Check sheet for the modelled part. Datum: model origin and axes. Units: mm. Face numbers are marked on the shaded views. Give positions to 0.01 mm unless a question says otherwise; leave off trailing zeros. Write each loop counter-clockwise with the first axis right and the second up, starting at its lowest first coordinate (ties: lowest second). Pieces come first, ordered by that corner, then holes.
from build123d import *

# Parameters (mm, degrees)
SKETCH1_W           = 105
SKETCH1_H           = 50
BOSS_EXTRUDE1_DEPTH = 5
BOSS_EXTRUDE2_DEPTH = 5


with BuildPart() as part:
    # Sketch1 → Boss-Extrude1 (new body)
    with BuildSketch(Plane(origin=(0, 0, 0), x_dir=(1, 0, 0), z_dir=(0, 1, 0))):
        Rectangle(SKETCH1_W, SKETCH1_H)
    extrude(amount=BOSS_EXTRUDE1_DEPTH)

    # Sketch2 → Boss-Extrude2 (add)
    with BuildSketch(Plane(origin=(0, 5, 0), x_dir=(1, 0, 0), z_dir=(0, 1, 0))):
        Polygon((-52.5, 25), (-52.5, -25), (52.5, -25), (52.5, 25), (47.5, 25), (47.5, -20), (-47.5, -20), (-47.5, 25), align=None)
    extrude(amount=BOSS_EXTRUDE2_DEPTH)


solid = part.part
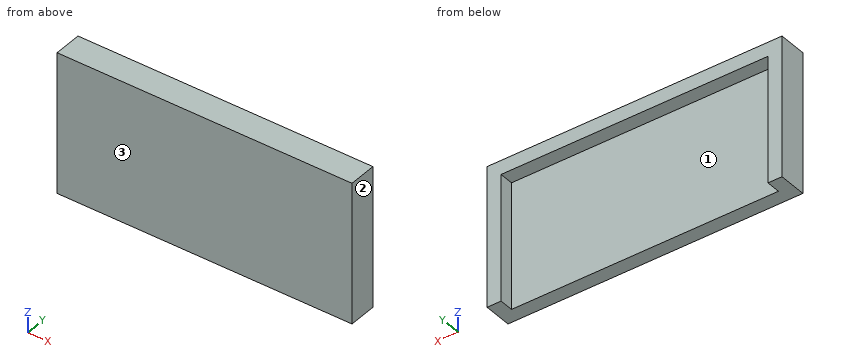
1) Draft check along X on the marked faces 1, 2 and 3. Enter one of: +X half, -X half, draft (parallel to the pull), parting line (faces both ways), or undercut.
2) Sectioned sample at B-B on y = 6. Record the boundary of the cut face in (x, z), then the cut area to 3 significant figures.
3) Scan lines: L1, parallel to X at y = 6, z = -5; L2, parallel to Z at x = -44, y = 6; L3, parallel to Y at x = 11.5, z = -15.5. Record each from-to range of solid material in increasing order.
4) Sectioned sample at C-C on x = 19. Record the boundary of the cut face in (y, z), then the cut area to 3 significant figures.
5) Gauge pin test, flat end, axial feed: pin 1 (13.5 mm diameter, centred on x = -15.5, z = -4.5, fed in from +Y). Record the tip position at first contact, or that the pin passes through.
6) Sectioned sample at A-A on z = -10.5. Record the boundary of the cut face in (x, y).
Answers below:
1. face 1: undercut
1. face 2: +X half
1. face 3: draft
2. outline: (-52.5, -25) - (-47.5, -25) - (-47.5, 20) - (47.5, 20) - (47.5, -25) - (52.5, -25) - (52.5, 25) - (-52.5, 25) - close
2. area: 975 mm2
3. L1: x = -52.5 to -47.5, 47.5 to 52.5
3. L2: z = 20 to 25
3. L3: y = 0 to 5
4. outline: (0, -25) - (5, -25) - (5, 20) - (10, 20) - (10, 25) - (0, 25) - close
4. area: 275 mm2
5. pin 1: stops at y = 5
6. outline: (-52.5, 0) - (52.5, 0) - (52.5, 10) - (47.5, 10) - (47.5, 5) - (-47.5, 5) - (-47.5, 10) - (-52.5, 10) - close
